from build123d import *

# Parameters (mm, degrees)
ESQUISSE1_W        = 10
ESQUISSE1_H        = 30
ESQUISSE1_R        = 2.6
BOSS_EXTRU_1_DEPTH = 5
ESQUISSE2_W        = 2
ESQUISSE2_H        = 30
BOSS_EXTRU_2_DEPTH = 5
CONG_1_R           = 5


with BuildPart() as part:
    # Esquisse1 → Boss.-Extru.1 (new body)
    with BuildSketch(Plane.XY):
        with Locations((40, -67.25)):
            Rectangle(ESQUISSE1_W, ESQUISSE1_H)
        with Locations((40, -77.25)):
            Circle(ESQUISSE1_R, mode=Mode.SUBTRACT)
        with Locations((40, -57.25)):
            Circle(ESQUISSE1_R, mode=Mode.SUBTRACT)
    extrude(amount=BOSS_EXTRU_1_DEPTH)

    # Esquisse2 → Boss.-Extru.2 (add)
    with BuildSketch(Plane(origin=(45, 0, 0), x_dir=(0, 0, -1), z_dir=(1, 0, 0))):
        with Locations((-4, -67.25)):
            Rectangle(ESQUISSE2_W, ESQUISSE2_H)
    extrude(amount=BOSS_EXTRU_2_DEPTH)

    # Congé1
    cong_1_edges = [part.edges().sort_by_distance(p)[0] for p in [
        (50, -82.25, 4),
        (50, -52.25, 4),
        (35, -52.25, 2.5),
        (35, -82.25, 2.5),
    ]]
    fillet(cong_1_edges, radius=CONG_1_R)


solid = part.part
The listing builds one solid part. Answer for the finished solid, in the listing's coordinates (mm). A direction names the side the tool comes from. Round coordinates to 2 decimals unless told otherwise and drop trailing zeros. Write each loop counter-clockwise with the first axis right and the second up, starting at its lowest first coordinate (ties: lowest second). Pieces come first, ordered by that corner, then holes. Notation, with made-up numbers: (-16.5, 43) - (15.5, 43) arc R33 cw to (15.5, 80) - close; hole circle Ø10 at (7, 19.5). An arc over 180 degrees is marked (long way). Use a Markdown table: item, result. Add a question column.
1. The part is cut by section B-B (y = -56.25). Write down the section's boundary in (x, z), and give its area (3 significant figures).
2. For a pull along Y with two mould halves and no side action, classify faces 1 (the face through (47, -67, 3)), 2 (the face through (39.662, -74.672, 2.465)), 3 (the face through (48.5, -80.82, 3.99)) as +Y half, -Y half, draft (parallel to the pull), parting line (faces both ways), or undercut.
3. Consider line 1 (Y direction, x = 40, z = 2.8); line 2 (Y direction, x = 38.5, z = 4.2); line 3 (X direction, y = -65.5, z = 1.2). Determine where each line is inside the solid, lowest interval first.
4. A tool of negligible diameter and unlimited length cuts with its end or side. For faces 4 (the face through (35, -67, 2)), 5 (the face through (45, -67, 1)), from which of +Z, -Z, +X, -X, +Y, -Y can it reach the whole face along a straight path? Write none if from no direction.
5. The part is cut by section C-C (x = 39.5). Write down the section's boundary in (y, z), and give its area (3 significant figures).
6. The part is cut by section A-A (z = 4.4). Write down the section's boundary in (x, y).
7. The part is cut by section D-D (z = 0.7). Write down the section's boundary in (x, y), and give its area (3 significant figures).
8. Flat-ended cylindrical pins translate along their axes: P1, Ø1.5, axis at y = -66.5, z = 1.5, coming from the +X side; P2, Ø5.5, axis at x = 46.5, y = -72, coming from the -Z side. Find the tip coordinate at first contact, or state that the pin passes through.
Reported:
| question | item | result |
|---|---|---|
| 1 | outline | (35.1, 0) - (37.6, 0) - (37.6, 5) - (35.1, 5) - close; (42.4, 0) - (45, 0) - (45, 3) - (49.9, 3) - (49.9, 5) - (42.4, 5) - close |
| 1 | area | 35.3 mm^2 |
| 2 | face 1 | draft |
| 2 | face 2 | undercut |
| 2 | face 3 | -Y half |
| 3 | line 1 | -82.25 to -79.85, -74.65 to -59.85, -54.65 to -52.25 |
| 3 | line 2 | -82.02 to -79.37, -75.13 to -59.37, -55.13 to -52.48 |
| 3 | line 3 | 35 to 45 |
| 4 | face 4 | +Z, -Z, -X, +Y, -Y |
| 4 | face 5 | -Z, +X, +Y, -Y |
| 5 | outline | (-82.22, 0) - (-79.8, 0) - (-79.8, 5) - (-82.22, 5) - close; (-74.7, 0) - (-59.8, 0) - (-59.8, 5) - (-74.7, 5) - close; (-54.7, 0) - (-52.28, 0) - (-52.28, 5) - (-54.7, 5) - close |
| 5 | area | 98.7 mm^2 |
| 6 | outline | (35, -77.25) arc R5 ccw to (40, -82.25) - (45, -82.25) arc R5 ccw to (50, -77.25) - (50, -57.25) arc R5 ccw to (45, -52.25) - (40, -52.25) arc R5 ccw to (35, -57.25) - close; hole circle Ø5.2 at (40, -77.25); hole circle Ø5.2 at (40, -57.25) |
| 7 | outline | (35, -77.25) arc R5 ccw to (40, -82.25) - (45, -82.25) - (45, -52.25) - (40, -52.25) arc R5 ccw to (35, -57.25) - close; hole circle Ø5.2 at (40, -77.25); hole circle Ø5.2 at (40, -57.25) |
| 7 | area | 247 mm^2 |
| 8 | P1 | x = 45 |
| 8 | P2 | z = 0 |
